from build123d import *

# Parameters (mm, degrees)
EXTRUDE_1_DEPTH = 25
FILLET_1_R      = 10
FILLET_2_R      = 10
FILLET_3_R      = 10
FILLET_4_R      = 10


with BuildPart() as part:
    # Эскиз1 → Вытянуть1 (new body)
    with BuildSketch(Plane(origin=(0, 0, 0), x_dir=(1, 0, 0), z_dir=(0, 1, 0))):
        with BuildLine():
            Line((67.101671661, -51.500497432), (112.378503317, -51.500497432))
            ThreePointArc((112.378503317, -51.500497432), (136.559037069, -53.030762447), (112.368799134, -54.399087045))
            Line((112.368799134, -54.399087045), (67.191980368, -53.918527595))
            ThreePointArc((67.191980368, -53.918527595), (1.146798105, -55.174484728), (67.101671661, -51.500497432))
        make_face()
        with BuildLine():
            Line((65.623717724, -52.474815373), (113.434997223, -52.474815373))
            ThreePointArc((113.434997223, -52.474815373), (135.422626362, -53.070517379), (113.428639384, -53.344803486))
            Line((113.428639384, -53.344803486), (65.65222177, -53.344262878))
            ThreePointArc((65.65222177, -53.344262878), (2.674800085, -54.973729362), (65.623717724, -52.474815373))
        make_face(mode=Mode.SUBTRACT)
    extrude(amount=EXTRUDE_1_DEPTH)

    # Скругление1
    fillet_1_edges = [part.edges().sort_by_distance(p)[0] for p in [
        (67.191980368, 12.5, 53.918527595),
    ]]
    fillet(fillet_1_edges, radius=FILLET_1_R)

    # Скругление2
    fillet_2_edges = [part.edges().sort_by_distance(p)[0] for p in [
        (65.65222177, 12.5, 53.344262878),
    ]]
    fillet(fillet_2_edges, radius=FILLET_2_R)

    # Скругление3
    fillet_3_edges = [part.edges().sort_by_distance(p)[0] for p in [
        (65.623717724, 12.5, 52.474815373),
        (67.101671661, 12.5, 51.500497432),
    ]]
    fillet(fillet_3_edges, radius=FILLET_3_R)

    # Скругление4
    fillet_4_edges = [part.edges().sort_by_distance(p)[0] for p in [
        (113.428639384, 12.5, 53.344803486),
        (113.434997223, 12.5, 52.474815373),
        (112.378503317, 12.5, 51.500497432),
        (112.368799134, 12.5, 54.399087045),
    ]]
    fillet(fillet_4_edges, radius=FILLET_4_R)


solid = part.part
Part model, mm, in its own coordinate system. A direction names the side the tool comes from. Give positions to 0.01 mm unless a question says otherwise; leave off trailing zeros. Write each loop counter-clockwise with the first axis right and the second up, starting at its lowest first coordinate (ties: lowest second). Pieces come first, ordered by that corner, then holes.
1) Probe L1, parallel to Z at x = 125, y = 21.75; L2, parallel to X at y = 18.5, z = 45.5; L3, parallel to X at y = 15.5, z = 57.5. List the from-to ranges inside material, lowest first.
Resolved:
L1: z = 40.87 to 42.01, 63.97 to 65.11
L2: x = 2.22 to 3.81, 64.51 to 66.19, 114.87 to 116.37, 132.48 to 133.97
L3: x = 1.32 to 2.86, 66.46 to 68.41, 112.72 to 114.27, 134.46 to 135.69
2) Two-plate mould, pull along X, no slides. Class faces 5 (the face through (90, 12, 51.5)), 6 (the face through (69, 0, 56)): released by +X, released by -X, zero draft, split by the parting line, or undercut.
Resolved:
face 5: undercut
face 6: zero draft
3) Cut at A-A on y = 12.75. Write the cut outline in (x, z).
Resolved:
outline: (65.78, 44.39) arc R10 cw to (75.35, 51.5) - (105.5, 51.5) arc R10 cw to (114.05, 46.69) arc R12.14 ccw (long way) to (114, 59.2) arc R10 cw to (105.52, 54.33) - (76.1, 54.01) arc R10 cw to (66.27, 61.67) arc R33.03 ccw (long way) to start; hole (64.43, 45.24) arc R10 cw to (74.04, 52.47) - (106.25, 52.47) arc R10 cw to (114.9, 47.48) arc R11 ccw (long way) to (114.85, 58.41) arc R10 cw to (106.15, 53.34) - (74.58, 53.34) arc R10 cw to (64.84, 61.08) arc R31.5 ccw (long way) to start
4) Which spindle directions (+Z, -Z, +X, -X, +Y, -Y) get a long thin tool onto all of the face, cutting with end or side? Do faces 1 (the face through (110.33, 12.68, 55.62)), 2 (the face through (69, 25, 56)), 3 (the face through (110.343, 12.675, 50.251)), 4 (the face through (111.124, 12.675, 54.668)). Say none if no direction does.
Resolved:
face 1: +Z, +Y, -Y
face 2: +Z, -Z, +X, -X, +Y
face 3: -Z, +Y, -Y
face 4: +Y, -Y
5) Pin check, flat tips, straight feed: pin 1 (3 mm diameter, centred on y = 6.5, z = 43, fed in from -X); pin 2 (12.5 mm diameter, centred on x = 93, y = 17, fed in from -Z); pin 3 (5 mm diameter, centred on x = 46, y = 9.5, fed in from -Z). Stop position of each tip, or through.
Resolved:
pin 1: stops at x = 2.5
pin 2: stops at z = 51.5
pin 3: stops at z = 22.26
6) Cut at C-C on x = 19. Write the cut outline in (y, z), then the cut area to 3 significant figures.
Resolved:
outline: (0, 24.59) - (25, 24.59) - (25, 26.33) - (0, 26.33) - close; (0, 81.55) - (25, 81.55) - (25, 83.29) - (0, 83.29) - close
area: 86.9 mm2
7) Cut at B-B on z = 72.5. Write the cut outline in (x, y), then the cut area to 3 significant figures.
Resolved:
outline: (6.83, 0) - (8.71, 0) - (8.71, 25) - (6.83, 25) - close; (59.61, 0) - (61.49, 0) - (61.49, 25) - (59.61, 25) - close
area: 93.8 mm2
